Part model, mm, in its own coordinate system. A direction names the side the tool comes from. Round coordinates to 2 decimals unless told otherwise and drop trailing zeros. Write each loop counter-clockwise with the first axis right and the second up, starting at its lowest first coordinate (ties: lowest second). Pieces come first, ordered by that corner, then holes. Notation, with made-up numbers: M 83,-17 L 118,-17 A31 cw 118,18 Z; hole C 19,47 d4. An arc over 180 degrees is marked long. Answer as a JSON object with one key per item and string values. Group by question number.
1. Which spindle directions (+Z, -Z, +X, -X, +Y, -Y) get a long thin tool onto all of the face, cutting with end or side? Do faces 1 (the face through (-5, 21, 3)), 2 (the face through (0, -22, 2)), 3 (the face through (4.029, 12, 7)). Say none if no direction does.
2. Band-saw the part on C-C, the plane z = 5.5. Count the separate pieces of the cut face and the enclosed holes in it, plus the area to 3 significant figures.
3. Band-saw the part on D-D, the plane x = 3.5. Write the cut outline in (y, z), plus the area to 3 significant figures.
4. Drill centre lines: line 1 (X direction, y = 7, z = 3); line 2 (X direction, y = -12, z = 11.5); line 3 (X direction, y = 18, z = 3.75). Where is each one in solid material? Low to high. Write a range as from..to.
5. Band-saw the part on A-A, the plane x = -8.75. Write the cut outline in (y, z), plus the area to 3 significant figures.
6. Drop flat-ended pins along their axis: pin 1 (3 mm diameter, centred on x = -10, z = 10, fed in from -Y); pin 2 (9.5 mm diameter, centred on x = 7.5, y = 14, fed in from -Z); pin 3 (1.6 mm diameter, centred on y = 21.5, z = 8, fed in from +X). Give the stop position or say it passes through.
7. Two-plate mould, pull along Z, no slides. Class faces 4 (the face through (-13, 2, 0)), 5 (the face through (-14.18, -21.4, 1.67)), 6 (the face through (-14, 15, 3)): +Z half, -Z half, draft (parallel to the pull), parting line (faces both ways), or undercut.
8. Band-saw the part on B-B, the plane y = -9. Write the cut outline in (x, z).
from build123d import *
from OCP.BRepFilletAPI import BRepFilletAPI_MakeChamfer

# Parameters (mm, degrees)
SKETCH1_W           = 29.5
SKETCH1_H           = 44
SKETCH1_W_2         = 25.5
SKETCH1_H_2         = 40
BOSS_EXTRUDE1_DEPTH = 12
BOSS_EXTRUDE2_START = 12
SKETCH1_2_W         = 29.5
SKETCH1_2_H         = 44
SKETCH1_2_W_2       = 25.5
SKETCH1_2_H_2       = 40
BOSS_EXTRUDE2_DEPTH = 2
BOSS_EXTRUDE3_DEPTH = 10.4
CUT_EXTRUDE1_REACH  = 50.472
SKETCH3_W           = 14.779376432
SKETCH3_H           = 9
CUT_EXTRUDE2_REACH  = 41.373
SKETCH4_W           = 9
SKETCH4_H           = 10.467816728
FILLET1_R           = 2
FILLET2_SIZE        = 8
FILLET2_SIZE2       = 10
SKETCH6_R           = 2
CUT_EXTRUDE3_DEPTH  = 8.4
FILLET3_R           = 5
FILLET5_R           = 2
FILLET6_R           = 2


with BuildPart() as part:
    # Sketch1 → Boss-Extrude1 (new body)
    with BuildSketch(Plane.XY):
        Rectangle(SKETCH1_W, SKETCH1_H)
        Rectangle(SKETCH1_W_2, SKETCH1_H_2, mode=Mode.SUBTRACT)
    extrude(amount=BOSS_EXTRUDE1_DEPTH)

    # Sketch1<2> → Boss-Extrude2 (add)
    # profile 1 of 2: a face of its own
    with BuildSketch(Plane.XY.offset(BOSS_EXTRUDE2_START)):
        Rectangle(SKETCH1_2_W, SKETCH1_2_H)
        Rectangle(SKETCH1_2_W_2, SKETCH1_2_H_2, mode=Mode.SUBTRACT)
    # profile 2 of 2: a face of its own
    with BuildSketch(Plane.XY.offset(BOSS_EXTRUDE2_START)):
        Rectangle(SKETCH1_2_W_2, SKETCH1_2_H_2)
    extrude(amount=BOSS_EXTRUDE2_DEPTH)

    # Sketch2 → Boss-Extrude3 (add)
    with BuildSketch(Plane(origin=(0, 0, 12), x_dir=(-1, 0, 0), z_dir=(0, 0, -1))):
        Polygon((-4.029376432, 20), (-4.029376432, 4.682180434), (-12.75, 4.682180434), (-12.75, -4.051886914), (-2.029376432, -4.051886914), (-2.029376432, 20), align=None)
    extrude(amount=BOSS_EXTRUDE3_DEPTH)

    # Sketch3 → Cut-Extrude1 (cut, up to next)
    with BuildSketch(Plane(origin=(0, 22, 0), x_dir=(1, 0, 0), z_dir=(0, 1, 0)), mode=Mode.PRIVATE) as cut_extrude1_sk1:
        with Locations((-5.360311784, -7.5)):
            Rectangle(SKETCH3_W, SKETCH3_H)
    cut_extrude1_tool1 = extrude(cut_extrude1_sk1.sketch, amount=-CUT_EXTRUDE1_REACH, mode=Mode.PRIVATE) & part.part
    add(cut_extrude1_tool1.solids().sort_by_distance((-5.360312, 22, 7.5))[0], mode=Mode.SUBTRACT)

    # Sketch4 → Cut-Extrude2 (cut, up to next)
    with BuildSketch(Plane.ZY.offset(14.75), mode=Mode.PRIVATE) as cut_extrude2_sk1:
        with Locations((7.5, 14.766091636)):
            Rectangle(SKETCH4_W, SKETCH4_H)
    cut_extrude2_tool1 = extrude(cut_extrude2_sk1.sketch, amount=-CUT_EXTRUDE2_REACH, mode=Mode.PRIVATE) & part.part
    add(cut_extrude2_tool1.solids().sort_by_distance((-14.75, 14.766092, 7.5))[0], mode=Mode.SUBTRACT)

    # Fillet1
    fillet1_edges = [part.edges().sort_by_distance(p)[0] for p in [
        (-14.75, 22, 7),
        (14.75, 22, 7),
    ]]
    fillet(fillet1_edges, radius=FILLET1_R - 0.0001)  # a hair under: the kernel refuses the full size

    # Fillet2: one chamfer whose edges measure the first distance from different faces: ONE call of the kernel's chamfer builder (chamfer() names one face for all edges)
    fillet2_edges_1 = [part.edges().sort_by_distance(p)[0] for p in [
        (0, -20, 12),
    ]]
    fillet2_side_1 = [part.faces().sort_by_distance(p)[0] for p in [
        (-2.893950715, -1.385908374, 12),
    ]]
    fillet2_edges_2 = [part.edges().sort_by_distance(p)[0] for p in [
        (0, -22, 14),
    ]]
    fillet2_side_2 = [part.faces().sort_by_distance(p)[0] for p in [
        (0, -0.028542601, 14),
    ]]
    fillet2 = BRepFilletAPI_MakeChamfer(part.part.solid().wrapped)
    for e in fillet2_edges_1:
        fillet2.Add(FILLET2_SIZE, FILLET2_SIZE2, e.wrapped, fillet2_side_1[0].wrapped)  # the first distance lies on this face
    for e in fillet2_edges_2:
        fillet2.Add(FILLET2_SIZE, FILLET2_SIZE2, e.wrapped, fillet2_side_2[0].wrapped)  # the first distance lies on this face
    add(Compound.cast(fillet2.Shape()), mode=Mode.REPLACE)

    # Sketch6 → Cut-Extrude3 (cut)
    with BuildSketch(Plane(origin=(0, 0, 1.6), x_dir=(-1, 0, 0), z_dir=(0, 0, -1))):
        with Locations((-7.7635572, 0)):
            Circle(SKETCH6_R)
    extrude(amount=-CUT_EXTRUDE3_DEPTH, mode=Mode.SUBTRACT)

    # Fillet3
    fillet3_edges = [part.edges().sort_by_distance(p)[0] for p in [
        (2.029376432, -4.051886914, 6.8),
    ]]
    fillet(fillet3_edges, radius=FILLET3_R)

    # Fillet5
    fillet5_edges = [part.edges().sort_by_distance(p)[0] for p in [
        (0, -22, 4),
    ]]
    fillet(fillet5_edges, radius=FILLET5_R)

    # Fillet6
    fillet6_edges = [part.edges().sort_by_distance(p)[0] for p in [
        (14.75, -17.780868809, 9.273913988),
        (14.75, -22, 1.649218941),
        (-14.75, -22, 1.649218941),
        (-14.75, -17.780868809, 9.273913988),
        (-14.75, -21.887256638, 3.960451764),
        (14.75, -21.887256638, 3.960451764),
    ]]
    fillet(fillet6_edges, radius=FILLET6_R)


solid = part.part
Worked answers:
{
 "1": {"face 1": "+Y", "face 2": "+Z, -Z, +X, -X, -Y", "face 3": "-Z"},
 "2": {"separate pieces": "2", "enclosed holes": "2", "area": "366 mm^2"},
 "3": {"outline": "M -22,0 L -20,0 L -20,2 L -12,12 L -2.59,12 L -2.59,1.6 L 20,1.6 L 20,0 L 22,0 L 22,14 L -14,14 L -21.56,4.55 A2 ccw -22,3.3 Z", "area": "371 mm^2"},
 "4": {"line 1": "x = -14.75..-12.75, 2.03..4.03, 12.75..14.75", "line 2": "x = -14.75..-12.75, 12.75..14.75", "line 3": "x = 2.03..4.03, 12.75..14.75"},
 "5": {"outline": "M -22,0 L -20,0 L -20,2 L -12,12 L 22,12 L 22,14 L -14,14 L -21.56,4.55 A2 ccw -22,3.3 Z; M 20,0 L 22,0 L 22,3 L 20,3 Z", "area": "118 mm^2"},
 "6": {"pin 1": "stops at y = -18.4", "pin 2": "stops at z = 1.6", "pin 3": "stops at x = 14.62"},
 "7": {"face 4": "-Z half", "face 5": "draft", "face 6": "undercut"},
 "8": {"outline": "M -14.75,0 L -12.75,0 L -12.75,12 L 12.75,12 L 12.75,0 L 14.75,0 L 14.75,14 L -14.75,14 Z"}
}
